Verification items for this drawing (mm, ordinates from the low corner). A direction names the side the tool comes from. Give positions to 0.01 mm unless a question says otherwise; leave off trailing zeros. Write each loop counter-clockwise with the first axis right and the second up, starting at its lowest first coordinate (ties: lowest second). Pieces come first, ordered by that corner, then holes. Notation, with made-up numbers: (62.5, 20.25) -> (79.5, 20.25) arc R24 ccw to (79.5, 31.25) -> close; hole circle Ø2 at (-16, 18). An arc over 180 degrees is marked (long way). Write item = value, one per line.
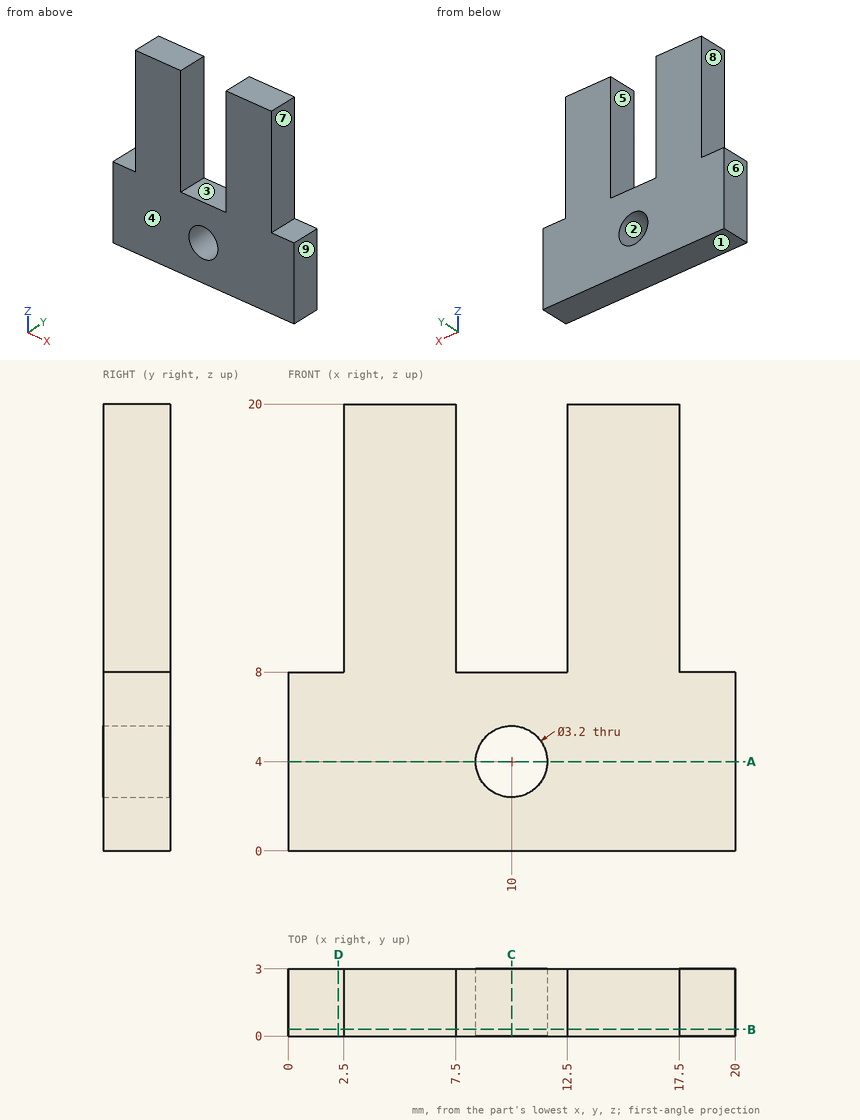
Item 1: Sectioned sample at B-B on y = 0.3. Record the cut outline in (x, z), then the cut area to 3 significant figures.
Response values:
outline = (0, 0) -> (20, 0) -> (20, 8) -> (17.5, 8) -> (17.5, 20) -> (12.5, 20) -> (12.5, 8) -> (7.5, 8) -> (7.5, 20) -> (2.5, 20) -> (2.5, 8) -> (0, 8) -> close; hole circle Ø3.2 at (10, 4)
area = 272 mm^2
Item 2: Sectioned sample at C-C on x = 10. Record the cut outline in (y, z), then the cut area to 3 significant figures.
Response values:
outline = (0, 0) -> (3, 0) -> (3, 2.4) -> (0, 2.4) -> close; (0, 5.6) -> (3, 5.6) -> (3, 8) -> (0, 8) -> close
area = 14.4 mm^2
Item 3: Set-up check for the marked faces 5, 6, 7, 8 and 9: record each of +Z, -Z, +X, -X, +Y, -Y from which the full face is reachable in a straight line by a thin tool's end or side.
Response values:
face_5 = +Z, +Y, -Y
face_6 = +Z, -Z, -X, +Y, -Y
face_7 = +Z, +X, +Y, -Y
face_8 = +Z, -X, +Y, -Y
face_9 = +Z, -Z, +X, +Y, -Y
Item 4: Sectioned sample at A-A on z = 4. Record the cut outline in (x, y), then the cut area to 3 significant figures.
Response values:
outline = (0, 0) -> (8.4, 0) -> (8.4, 3) -> (0, 3) -> close; (11.6, 0) -> (20, 0) -> (20, 3) -> (11.6, 3) -> close
area = 50.4 mm^2
Item 5: Mould release check, pull along Z, two halves, no side actions. Record for the marked faces 1, 2, 3 and 4: +Z half, -Z half, draft (parallel to the pull), parting line (faces both ways), or undercut.
Response values:
face_1 = -Z half
face_2 = undercut
face_3 = +Z half
face_4 = draft
Item 6: Material ranges on line 1 (X direction, y = 2.2, z = 13.75); line 2 (Z direction, x = 10, y = 1.85); line 3 (X direction, y = 2.2, z = 4), recorded low to high.
Response values:
line_1 = 2.5 to 7.5, 12.5 to 17.5
line_2 = 0 to 2.4, 5.6 to 8
line_3 = 0 to 8.4, 11.6 to 20
Item 7: Go/stop test with flat-tipped pins: P1, Ø1.5, axis at y = 1.5, z = 13.5, coming from the +X side; P2, Ø0.9, axis at y = 1.5, z = 15, coming from the -X side. Record where each tip stops, or that it passes through.
Response values:
P1 = 17.5
P2 = 2.5
Item 8: Sectioned sample at D-D on x = 2.25. Record the cut outline in (y, z).
Response values:
outline = (0, 0) -> (3, 0) -> (3, 8) -> (0, 8) -> close
